The listing builds one solid part. Answer for the finished solid, in the listing's coordinates (mm). A direction names the side the tool comes from. Round coordinates to 2 decimals unless told otherwise and drop trailing zeros. Loops run counter-clockwise (first coordinate to the right, second up) from the corner with the lowest first, then second, coordinate; pieces in that order, holes last. Notation, with made-up numbers: (73, 61.25) - (108, 61.25) arc R18 cw to (108, 95.25) - close; hole circle Ø4 at (61.25, 74.5). An arc over 180 degrees is marked (long way). One line per item, written item: value.
```python
from build123d import *

# Parameters (mm, degrees)
SKETCH1_R           = 15
SKETCH1_W           = 15
SKETCH1_H           = 15
BOSS_EXTRUDE1_DEPTH = 15
SKETCH2_R           = 15
BOSS_EXTRUDE2_DEPTH = 5
BOSS_EXTRUDE3_DEPTH = 20
FILLET1_R           = 3


with BuildPart() as part:
    # Sketch1 → Boss-Extrude1 (new body)
    with BuildSketch(Plane(origin=(0, 0, 0), x_dir=(1, 0, 0), z_dir=(0, 1, 0))):
        with Locations(Location((0, 0, 0), (0, 0, 270))):
            Circle(SKETCH1_R)
        Rectangle(SKETCH1_W, SKETCH1_H, mode=Mode.SUBTRACT)
    extrude(amount=BOSS_EXTRUDE1_DEPTH)

    # Sketch2 → Boss-Extrude2 (add)
    with BuildSketch(Plane(origin=(0, 15, 0), x_dir=(1, 0, 0), z_dir=(0, 1, 0))):
        with Locations(Location((0, 0, 0), (0, 0, 270))):
            Circle(SKETCH2_R)
    extrude(amount=BOSS_EXTRUDE2_DEPTH)

    # Sketch3 → Boss-Extrude3 (add)
    with BuildSketch(Plane(origin=(0, 20, 0), x_dir=(1, 0, 0), z_dir=(0, 1, 0))):
        Polygon((2.5, -1.443375673), (2.5, 1.443375673), (0, 2.886751346), (-2.5, 1.443375673), (-2.5, -1.443375673), (0, -2.886751346), align=None)
    extrude(amount=BOSS_EXTRUDE3_DEPTH)

    # Fillet1
    fillet1_edges = [part.edges().sort_by_distance(p)[0] for p in [
        (2.5, 20, 0),
        (1.25, 20, -2.165063509),
        (-1.25, 20, -2.165063509),
        (-2.5, 20, 0),
        (-1.25, 20, 2.165063509),
        (1.25, 20, 2.165063509),
    ]]
    fillet(fillet1_edges, radius=FILLET1_R)


solid = part.part
```
1) For faces 4 (the flat face through (7.5, 7, 0)), 5 (the flat face through (-2.5, 31, 0)), 6 (the flat face through (1.267, 31.381, -2.155)), determine the directions among +Z, -Z, +X, -X, +Y, -Y from which every point of the face is accessible in a straight line to the end or side of a thin tool.
Final values:
face 4: -Y
face 5: +Z, -Z, -X, +Y
face 6: -Z, +X, +Y
2) Consider L1, parallel to Y at x = 11.25, z = -5.75; L2, parallel to Y at x = -6.5, z = 1; L3, parallel to Z at x = -4.75, y = 9.5. Determine where each line is inside the solid, lowest interval first.
Final values:
L1: 0 to 20
L2: 15 to 20
L3: -14.23 to -7.5, 7.5 to 14.23
3) A cutting plane is placed at A-A on y = 28. Give the vertices of the cut face in (x, z), and give its area (3 significant figures).
Final values:
outline: (-2.5, -1.44) - (0, -2.89) - (2.5, -1.44) - (2.5, 1.44) - (0, 2.89) - (-2.5, 1.44) - close
area: 21.7 mm2
4) Each of these flat-tipped pins is pushed along its axis until it touches: pin 1 Ø16.5 at (x, y) = (-1, 8.5) entering from -Z; pin 2 Ø2 at (x, y) = (4.5, 7) entering from -Z; pin 3 Ø5 at (x, y) = (8.5, 8.5) entering from -Z; pin 4 Ø1.5 at (y, z) = (18, -6.5) entering from -X. Where does it stop, or does it pass through?
Final values:
pin 1: z = -15
pin 2: z = -14.59
pin 3: z = -13.75
pin 4: x = -13.85
5) A cutting plane is placed at B-B on z = 0. Give the vertices of the cut face in (x, y), and give its area (3 significant figures).
Final values:
outline: (-15, 0) - (-7.5, 0) - (-7.5, 15) - (7.5, 15) - (7.5, 0) - (15, 0) - (15, 20) - (5.5, 20) arc R3 cw to (2.5, 23) - (2.5, 40) - (-2.5, 40) - (-2.5, 23) arc R3 cw to (-5.5, 20) - (-15, 20) - close
area: 479 mm2
6) A cutting plane is placed at D-D on y = 22.5. Give the vertices of the cut face in (x, z).
Final values:
outline: (-2.54, -1.47) - (0, -2.94) - (2.54, -1.47) - (2.54, 1.47) - (0, 2.94) - (-2.54, 1.47) - close
7) A cutting plane is placed at C-C on x = 6.75. Give the vertices of the cut face in (y, z), and give its area (3 significant figures).
Final values:
outline: (0, -13.4) - (20, -13.4) - (20, 13.4) - (0, 13.4) - (0, 7.5) - (15, 7.5) - (15, -7.5) - (0, -7.5) - close
area: 311 mm2
8) For a pull along X with two mould halves and no side action, classify faces 1 (the cylindrical face through (-3.81, 20.52, 0.04)), 2 (the flat face through (1.233, 31.381, 2.175)), 3 (the flat face through (0, 15, 0)) as released by +X, released by -X, zero draft, split by the parting line, or undercut.
Final values:
face 1: released by -X
face 2: released by +X
face 3: undercut
